Geometry: final body of the model. Coordinates: model frame, mm. A direction names the side the tool comes from. Give positions to 0.01 mm unless a question says otherwise; leave off trailing zeros. Write each loop counter-clockwise with the first axis right and the second up, starting at its lowest first coordinate (ties: lowest second). Pieces come first, ordered by that corner, then holes. Notation, with made-up numbers: (16.5, 26) -> (67.5, 26) arc R27 ccw to (67.5, 64) -> close; hole circle Ø5 at (14.5, 63). An arc over 180 degrees is marked (long way). Answer as a JSON object with one key per item and string values. Group by question number.
(1) Section query A-A on y = 0. Output: boundary loops of the cut face in (x, z) (3 decimals), plus the area to 3 significant figures.
(2) Set-up query: faces 1 (the face through (-17.58, -1.57, 9.86)), 2 (the face through (-16, -9.45, 1)), 3 (the face through (16, 9.45, 1)), 4 (the face through (18, 0, 2.2)), 5 (the face through (-18, 0, 2.2)). Return all of +Z, -Z, +X, -X, +Y, -Y with unobstructed straight access to the full face (end or side cutting, diameter ignored); none if empty.
(3) Contact query for flat-ended pins moving along their axis: pin 1 Ø2.5 at (x, y) = (17.5, -4) entering from +Z; pin 2 Ø4 at (x, y) = (-17.5, 0.5) entering from +Z; pin 3 Ø1.8 at (x, z) = (16, 1) entering from -Y. Output: stop coordinate, or through.
(4) Material intervals for probe 1 along X at (y, z) = (0, 51.25); probe 2 along X at (y, z) = (-5, 53.5), sorted ascending.
(5) Section query D-D on z = 38. Output: boundary loops of the cut face in (x, y), plus the area to 3 significant figures.
(6) Section query C-C on z = 29. Output: boundary loops of the cut face in (x, y).
(7) Section query B-B on x = 0. Output: boundary loops of the cut face in (y, z).
from build123d import *

# Parameters (mm, degrees)
F1_DEPTH = 2.2
F2_DEPTH = 20
F4_R     = 9.25
F4_R_2   = 7
F5_DEPTH = 25
F8_SIZE2 = 5
F8_SIZE  = 0.5


with BuildPart() as f1:
    # F0 (on Top) → F1 (new body)
    with BuildSketch(Plane.XY):
        with BuildLine():
            ThreePointArc((-14.9070453142, -9.45), (-17.65, 0), (-14.9070453142, 9.45))
            Line((-14.9070453142, 9.45), (-17.5414687241, 9.45))
            ThreePointArc((-17.5414687241, 9.45), (-19.925, 0), (-17.5414687241, -9.45))
            Line((-17.5414687241, -9.45), (-14.9070453142, -9.45))
        make_face()
        with BuildLine():
            ThreePointArc((14.9070453142, 9.45), (16.9503960101, 4.9200177949), (17.65, 0))
            ThreePointArc((17.65, 0), (16.9503960101, -4.9200177949), (14.9070453142, -9.45))
            Line((14.9070453142, -9.45), (17.5414687241, -9.45))
            ThreePointArc((17.5414687241, -9.45), (19.925, 0), (17.5414687241, 9.45))
            Line((17.5414687241, 9.45), (14.9070453142, 9.45))
        make_face()
        with BuildLine():
            Line((12.286069347, 9.45), (14.9070453142, 9.45))
            ThreePointArc((14.9070453142, 9.45), (0, 17.65), (-14.9070453142, 9.45))
            Line((-14.9070453142, 9.45), (-12.286069347, 9.45))
            ThreePointArc((-12.286069347, 9.45), (0, 15.5), (12.286069347, 9.45))
        make_face()
        with BuildLine():
            Line((-12.286069347, 9.45), (-14.9070453142, 9.45))
            ThreePointArc((-14.9070453142, 9.45), (-17.65, 0), (-14.9070453142, -9.45))
            Line((-14.9070453142, -9.45), (-12.286069347, -9.45))
            ThreePointArc((-12.286069347, -9.45), (-15.5, 0), (-12.286069347, 9.45))
        make_face()
        with BuildLine():
            ThreePointArc((-14.9070453142, -9.45), (0, -17.65), (14.9070453142, -9.45))
            Line((14.9070453142, -9.45), (12.286069347, -9.45))
            ThreePointArc((12.286069347, -9.45), (0, -15.5), (-12.286069347, -9.45))
            Line((-12.286069347, -9.45), (-14.9070453142, -9.45))
        make_face()
        with BuildLine():
            ThreePointArc((14.9070453142, -9.45), (16.9503960101, -4.9200177949), (17.65, 0))
            ThreePointArc((17.65, 0), (16.9503960101, 4.9200177949), (14.9070453142, 9.45))
            Line((14.9070453142, 9.45), (12.286069347, 9.45))
            ThreePointArc((12.286069347, 9.45), (14.6745370434, 4.9907877695), (15.5, 0))
            ThreePointArc((15.5, 0), (14.6745370434, -4.9907877695), (12.286069347, -9.45))
            Line((12.286069347, -9.45), (14.9070453142, -9.45))
        make_face()
    extrude(amount=F1_DEPTH)

    # F0 (on Top) → F2 (join)
    with BuildSketch(Plane.XY):
        with BuildLine():
            Line((12.286069347, 9.45), (14.9070453142, 9.45))
            ThreePointArc((14.9070453142, 9.45), (0, 17.65), (-14.9070453142, 9.45))
            Line((-14.9070453142, 9.45), (-12.286069347, 9.45))
            ThreePointArc((-12.286069347, 9.45), (0, 15.5), (12.286069347, 9.45))
        make_face()
        with BuildLine():
            Line((-12.286069347, 9.45), (-14.9070453142, 9.45))
            ThreePointArc((-14.9070453142, 9.45), (-17.65, 0), (-14.9070453142, -9.45))
            Line((-14.9070453142, -9.45), (-12.286069347, -9.45))
            ThreePointArc((-12.286069347, -9.45), (-15.5, 0), (-12.286069347, 9.45))
        make_face()
        with BuildLine():
            ThreePointArc((-14.9070453142, -9.45), (0, -17.65), (14.9070453142, -9.45))
            Line((14.9070453142, -9.45), (12.286069347, -9.45))
            ThreePointArc((12.286069347, -9.45), (0, -15.5), (-12.286069347, -9.45))
            Line((-12.286069347, -9.45), (-14.9070453142, -9.45))
        make_face()
        with BuildLine():
            ThreePointArc((14.9070453142, -9.45), (16.9503960101, -4.9200177949), (17.65, 0))
            ThreePointArc((17.65, 0), (16.9503960101, 4.9200177949), (14.9070453142, 9.45))
            Line((14.9070453142, 9.45), (12.286069347, 9.45))
            ThreePointArc((12.286069347, 9.45), (14.6745370434, 4.9907877695), (15.5, 0))
            ThreePointArc((15.5, 0), (14.6745370434, -4.9907877695), (12.286069347, -9.45))
            Line((12.286069347, -9.45), (14.9070453142, -9.45))
        make_face()
    extrude(amount=F2_DEPTH)



with BuildPart() as f5:
    # F4 (on offset) → F5 (new body)
    with BuildSketch(Plane.XY.offset(35)):
        Circle(F4_R)
        Circle(F4_R_2, mode=Mode.SUBTRACT)
    extrude(amount=F5_DEPTH)


with BuildPart() as f1_1:
    add(f1.part)

    add(f5.part)  # F7 merges F5
    # F6 (on Right) → F7 (revolve)
    with BuildSketch(Plane.YZ):
        Polygon((-9.25, 35), (-17.65, 20), (-15.5, 20), (-7, 35), align=None)
    revolve(axis=Axis((0, 0, 18.8534432091), (0, 0, -1)))

    # F8
    f8_edges = [f1_1.edges().sort_by_distance(p)[0] for p in [
        (-9.25, 0, 60),
    ]]
    f8_side = f1_1.faces().sort_by_distance((-8.98837, 0, 60))[0]
    chamfer(f8_edges, length=F8_SIZE, length2=F8_SIZE2, reference=f8_side)


solid = f1_1.part
Answer list:
{
 "1": {"outline": "(-19.925, 0) -> (-15.5, 0) -> (-15.5, 20) -> (-7, 35) -> (-7, 60) -> (-8.75, 60) -> (-9.25, 55) -> (-9.25, 35) -> (-17.65, 20) -> (-17.65, 2.2) -> (-19.925, 2.2) -> close; (7, 35) -> (15.5, 20) -> (15.5, 0) -> (19.925, 0) -> (19.925, 2.2) -> (17.65, 2.2) -> (17.65, 20) -> (9.25, 35) -> (9.25, 55) -> (8.75, 60) -> (7, 60) -> close", "area": "272 mm2"},
 "2": {"face 1": "+Z", "face 2": "+Z, -Z, -X, -Y", "face 3": "+Z, -Z, +X, +Y", "face 4": "+Z, +X", "face 5": "+Z, -X"},
 "3": {"pin 1": "z = 21.69", "pin 2": "z = 23.83", "pin 3": "y = -9.45"},
 "4": {"probe 1": "-9.25 to -7, 7 to 9.25", "probe 2": "-7.78 to -4.9, 4.9 to 7.78"},
 "5": {"outline": "circle Ø18.5 at (0, 0); hole circle Ø14 at (0, 0)", "area": "115 mm2"},
 "6": {"outline": "circle Ø25.22 at (0, 0); hole circle Ø20.8 at (0, 0)"},
 "7": {"outline": "(-17.65, 0) -> (-15.5, 0) -> (-15.5, 20) -> (-7, 35) -> (-7, 60) -> (-8.75, 60) -> (-9.25, 55) -> (-9.25, 35) -> (-17.65, 20) -> close; (7, 35) -> (15.5, 20) -> (15.5, 0) -> (17.65, 0) -> (17.65, 20) -> (9.25, 35) -> (9.25, 55) -> (8.75, 60) -> (7, 60) -> close"}
}
